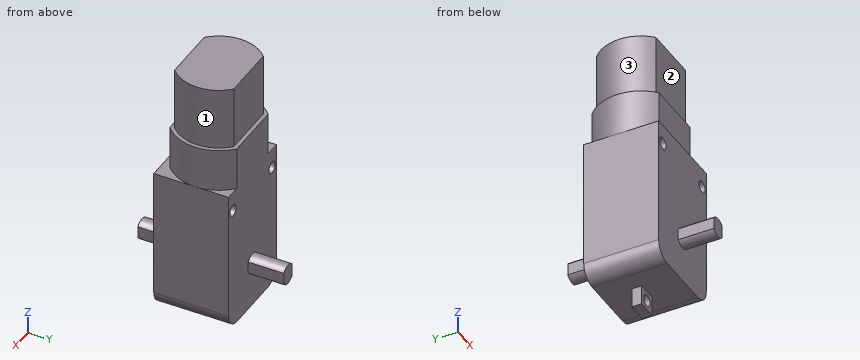
from build123d import *

# Parameters (mm, degrees)
SKETCH1_W           = 22.5
SKETCH1_H           = 19
BOSS_EXTRUDE1_DEPTH = 37
BOSS_EXTRUDE2_DEPTH = 11
BOSS_EXTRUDE3_DEPTH = 16
FILLET1_R           = 4
SKETCH6_W           = 5
SKETCH6_H           = 2.5
BOSS_EXTRUDE4_DEPTH = 5
SKETCH7_R           = 1.5
CUT_EXTRUDE1_DEPTH  = 5
SKETCH5_R           = 1.5
CUT_EXTRUDE3_DEPTH  = 19
BOSS_EXTRUDE5_DEPTH = 9
BOSS_EXTRUDE6_START = 9
BOSS_EXTRUDE6_DEPTH = 9


with BuildPart() as part:
    # Sketch1 → Boss-Extrude1 (new body)
    with BuildSketch(Plane.XY):
        Rectangle(SKETCH1_W, SKETCH1_H)
    extrude(amount=BOSS_EXTRUDE1_DEPTH)

    # Sketch3 → Boss-Extrude2 (add)
    with BuildSketch(Plane.XY.offset(37)):
        with BuildLine():
            Line((-7.369701486, -7.5), (7.369701486, -7.5))
            ThreePointArc((7.369701486, -7.5), (11.25, 1), (7.369701486, 9.5))
            Line((7.369701486, 9.5), (-7.369701486, 9.5))
            ThreePointArc((-7.369701486, 9.5), (-11.25, 1), (-7.369701486, -7.5))
        make_face()
    extrude(amount=BOSS_EXTRUDE2_DEPTH)

    # Sketch4 → Boss-Extrude3 (add)
    with BuildSketch(Plane.XY.offset(48)):
        with BuildLine():
            Line((5.23171695, 8.5), (-2.076174526, 8.5))
            Line((-2.076174526, 8.5), (-6.986594306, 8.5))
            ThreePointArc((-6.986594306, 8.5), (-10.25, 1), (-6.986594306, -6.5))
            Line((-6.986594306, -6.5), (-5.941237129, -6.5))
            Line((-5.941237129, -6.5), (4.647085632, -6.5))
            Line((4.647085632, -6.5), (6.986594306, -6.5))
            ThreePointArc((6.986594306, -6.5), (10.25, 1), (6.986594306, 8.5))
            Line((6.986594306, 8.5), (5.23171695, 8.5))
        make_face()
    extrude(amount=BOSS_EXTRUDE3_DEPTH)

    # Fillet1
    fillet1_edges = [part.edges().sort_by_distance(p)[0] for p in [
        (11.25, 0, 0),
        (-11.25, 0, 0),
    ]]
    fillet(fillet1_edges, radius=FILLET1_R)

    # Sketch6 → Boss-Extrude4 (add)
    with BuildSketch(Plane(origin=(0, 0, 0), x_dir=(-1, 0, 0), z_dir=(0, 0, -1))):
        with Locations((0.019167068, 0.75)):
            Rectangle(SKETCH6_W, SKETCH6_H)
    extrude(amount=BOSS_EXTRUDE4_DEPTH)

    # Sketch7 → Cut-Extrude1 (cut)
    with BuildSketch(Plane(origin=(0, 2, 0), x_dir=(1, 0, 0), z_dir=(0, 1, 0))):
        with Locations(Location((-0.009583534, 2.5, 0), (0, 0, 180))):
            Circle(SKETCH7_R)
    extrude(amount=-CUT_EXTRUDE1_DEPTH, mode=Mode.SUBTRACT)

    # Sketch5 → Cut-Extrude3 (cut)
    with BuildSketch(Plane(origin=(0, 9.5, 0), x_dir=(1, 0, 0), z_dir=(0, 1, 0))):
        with Locations(Location((-9.25, -32, 0), (0, 0, 180))):
            Circle(SKETCH5_R)
        with Locations(Location((9.25, -32, 0), (0, 0, 180))):
            Circle(SKETCH5_R)
    extrude(amount=-CUT_EXTRUDE3_DEPTH, mode=Mode.SUBTRACT)

    # Sketch5_5 → Boss-Extrude5 (add)
    with BuildSketch(Plane(origin=(0, 9.5, 0), x_dir=(1, 0, 0), z_dir=(0, 1, 0))):
        with BuildLine():
            Line((-2, -10), (-2, -13))
            ThreePointArc((-2, -13), (0, -14), (2, -13))
            Line((2, -13), (2, -10))
            ThreePointArc((2, -10), (0, -9), (-2, -10))
        make_face()
    extrude(amount=BOSS_EXTRUDE5_DEPTH)

    # Sketch8 → Boss-Extrude6 (add)
    with BuildSketch(Plane.XZ.offset(9.5).offset(BOSS_EXTRUDE6_START)):
        with BuildLine():
            Line((-2, 13), (-2, 10))
            ThreePointArc((-2, 10), (0, 9), (2, 10))
            Line((2, 10), (2, 13))
            ThreePointArc((2, 13), (0, 14), (-2, 13))
        make_face()
    extrude(amount=-BOSS_EXTRUDE6_DEPTH)


solid = part.part
Input: part model. Units: mm. Frame: model coordinates. Face numbers are marked on the shaded views. A direction names the side the tool comes from. Give positions to 0.01 mm unless a question says otherwise; leave off trailing zeros. Write each loop counter-clockwise with the first axis right and the second up, starting at its lowest first coordinate (ties: lowest second). Pieces come first, ordered by that corner, then holes. Notation, with made-up numbers: (67, -15.75) -> (120, -15.75) arc R6 cw to (120, -6.75) -> close; hole circle Ø1 at (1, 70). An arc over 180 degrees is marked (long way). Use one line per item in the form item = value. Start each with the question number.
1) Ray query, probe 1 along Y at (x, z) = (5.75, 57.5); probe 2 along Y at (x, z) = (-8.5, 17); probe 3 along Z at (x, y) = (4.75, -9). Return the intervals inside material, ascending. Write a range as from..to.
2) Set-up query: the marked faces 1, 2 and 3. Return all of +Z, -Z, +X, -X, +Y, -Y with unobstructed straight access to the full face (end or side cutting, diameter ignored); none if empty.
3) Section query C-C on x = -4.5. Return the cut outline in (y, z).
4) Pin query (flat end, axial travel): pin 1 (4 mm diameter, centred on x = -1, z = 57, fed in from -Y); pin 2 (3.5 mm diameter, centred on y = 15.5, z = 11, fed in from +X); pin 3 (5 mm diameter, centred on x = 9.25, z = 32, fed in from +Y); pin 4 (2.5 mm diameter, centred on x = -0.01, z = -2.5, fed in from +Y). Return the tip coordinate at first contact, or that it passes through.
5) Section query A-A on z = 32. Return the cut outline in (x, y), then the cut area to 4 significant figures.
6) Section query D-D on x = -8.5. Return the cut outline in (y, z), then the cut area to 3 significant figures.
7) Section query B-B on y = 3.5. Return the cut outline in (x, z).
Outcome:
q1.probe_1 = -6.5..8.5
q1.probe_2 = -9.5..9.5
q1.probe_3 = 0..37
q2.face_1 = +Z, +X
q2.face_2 = +Z, +X, -X, -Y
q2.face_3 = +Z, -X
q3.outline = (-9.5, 0) -> (9.5, 0) -> (9.5, 48) -> (8.5, 48) -> (8.5, 64) -> (-6.5, 64) -> (-6.5, 48) -> (-7.5, 48) -> (-7.5, 37) -> (-9.5, 37) -> close
q4.pin_1 = -6.5
q4.pin_2 = 2
q4.pin_3 = 9.5
q4.pin_4 = through
q5.outline = (-11.25, -9.5) -> (-10.75, -9.5) -> (-10.75, 9.5) -> (-11.25, 9.5) -> close; (-7.75, -9.5) -> (7.75, -9.5) -> (7.75, 9.5) -> (-7.75, 9.5) -> close; (10.75, -9.5) -> (11.25, -9.5) -> (11.25, 9.5) -> (10.75, 9.5) -> close
q5.area = 313.5 mm^2
q6.outline = (-9.5, 0.2) -> (9.5, 0.2) -> (9.5, 30.7) -> (-9.5, 30.7) -> close; (-9.5, 33.3) -> (9.5, 33.3) -> (9.5, 37) -> (8.37, 37) -> (8.37, 48) -> (6.73, 48) -> (6.73, 64) -> (-4.73, 64) -> (-4.73, 48) -> (-6.37, 48) -> (-6.37, 37) -> (-9.5, 37) -> close
q6.area = 995 mm^2
q7.outline = (-11.25, 4) arc R4 ccw to (-7.25, 0) -> (7.25, 0) arc R4 ccw to (11.25, 4) -> (11.25, 37) -> (10.97, 37) -> (10.97, 48) -> (9.94, 48) -> (9.94, 64) -> (-9.94, 64) -> (-9.94, 48) -> (-10.97, 48) -> (-10.97, 37) -> (-11.25, 37) -> close; hole circle Ø3 at (-9.25, 32); hole circle Ø3 at (9.25, 32)
